Model file for the job. Use its own axes, mm. Face numbers are marked on the shaded views. A direction names the side the tool comes from. Coordinates: 2 decimals unless noted, no trailing zeros. Order: outer loops, then holes, each group sorted by start corner. A loop starts at its lowest first (then second) coordinate and runs counter-clockwise, first axis right, second up. Notation, with made-up numbers: (-40, 52) -> (12, 52) arc R32 cw to (12, 84) -> close; hole circle Ø7 at (13, -5). An arc over 180 degrees is marked (long way). Write item = value, one per line. Start each with the question number.
Q1. Flat gauge pins, fed straight in: pin 1 (1 mm diameter, centred on x = 1.07, y = -7.26, fed in from +Z); pin 2 (1.5 mm diameter, centred on y = -35.5, z = -5.5, fed in from -X); pin 3 (2 mm diameter, centred on y = -36, z = -13, fed in from +X); pin 4 (2.5 mm diameter, centred on x = 4, y = -40, fed in from +Z). Where does each tip first touch, or does it go through?
Q2. Cut at D-D, the plane x = -1.75. List the corners of the cut face in (y, z), plus the area to 3 significant figures.
Q3. Cut at C-C, the plane y = -31.5. List the corners of the cut face in (x, z), plus the area to 4 significant figures.
Q4. Cut at B-B, the plane z = -11.75. List the corners of the cut face in (x, y), plus the area to 3 significant figures.
Q5. Cut at A-A, the plane z = -3. List the corners of the cut face in (x, y), plus the area to 3 significant figures.
Q6. 3-axis set-ups, long thin cutter, end or side, ignore diameter. For the marked faces 1 and 2: which of +Z, -Z, +X, -X, +Y, -Y reach the whole face in a straight line?
Q7. Wall check: line 1 (X direction, y = -35.5, z = -6.25); line 2 (Y direction, x = 1, z = -3); line 3 (Y direction, x = 3.75, z = -13.5). Give the ranges that are in metal, low to high. Write a range as from..to.
from build123d import *

# Parameters (mm, degrees)
EXTRUDE_START                = -2
EXTRUDE_1_DEPTH              = 13
SKETCH_2_R                   = 11
CUT_EXTRUDE_1_DEPTH          = 5
SKETCH_3_R                   = 1.5
EXTRUDE_2_DEPTH              = 2
EXTRUDE_3_DEPTH              = 2
HOLE_WIZARD_M2_4_D           = 1.6
HOLE_WIZARD_M2_4_DEPTH       = 5.2
HOLE_WIZARD_M2_4_CSINK_D     = 2.05
HOLE_WIZARD_M2_4_CSINK_ANGLE = 90
HOLE_WIZARD_M2_4_TIP         = 0.480688495
HOLE_WIZARD_M2_5_D           = 1.6
HOLE_WIZARD_M2_5_DEPTH       = 5.2
HOLE_WIZARD_M2_5_CSINK_D     = 2.05
HOLE_WIZARD_M2_5_CSINK_ANGLE = 90
HOLE_WIZARD_M2_5_TIP         = 0.480688495


with BuildPart() as part:
    # 草图1 → 凸台-拉伸1 (new body)
    with BuildSketch(Plane.XY.offset(EXTRUDE_START)):
        with BuildLine():
            Line((2.570888862, -12.45291013), (-3.464101615, -2))
            Line((-3.464101615, -2), (-5.196152423, -3))
            Line((-5.196152423, -3), (1.320888862, -14.287846621))
            Line((1.320888862, -14.287846621), (1.320888862, -44.355557574))
            ThreePointArc((1.320888862, -44.355557574), (1.933218512, -44.007523283), (2.570888862, -43.708438024))
            Line((2.570888862, -43.708438024), (2.570888862, -12.45291013))
        make_face()
    extrude(amount=-EXTRUDE_1_DEPTH)

    # 草图2 → 切除-拉伸1 (cut)
    with BuildSketch(Plane(origin=(0, 0, -15), x_dir=(-1, 0, 0), z_dir=(0, 0, -1))):
        with Locations((-6.070888862, -52)):
            Circle(SKETCH_2_R)
    extrude(amount=-CUT_EXTRUDE_1_DEPTH, mode=Mode.SUBTRACT)

    # 草图3 → 凸台-拉伸2 (add)
    with BuildSketch(Plane(origin=(0, 0, -15), x_dir=(-1, 0, 0), z_dir=(0, 0, -1))):
        with Locations((-4.070888862, -39.661037321)):
            Circle(SKETCH_3_R)
        with BuildLine():
            Line((-2.570888862, -41.571673193), (-2.570888862, -39.661037321))
            ThreePointArc((-2.570888862, -39.661037321), (-3.098777733, -40.803403266), (-4.310888798, -41.141712853))
            ThreePointArc((-4.310888798, -41.141712853), (-3.432117057, -41.321194666), (-2.570888862, -41.571673193))
        make_face()
        with BuildLine():
            Line((-2.570888862, -39.661037321), (-2.570888862, -38.161037321))
            Line((-2.570888862, -38.161037321), (-4.070888862, -38.161037321))
            ThreePointArc((-4.070888862, -38.161037321), (-3.010228691, -38.600377149), (-2.570888862, -39.661037321))
        make_face()
    extrude(amount=-EXTRUDE_2_DEPTH)

    # 草图4 → 凸台-拉伸3 (add)
    with BuildSketch(Plane.XY.offset(-2)):
        with BuildLine():
            Line((0.320888862, -8.555795813), (2.570888862, -12.45291013))
            Line((2.570888862, -12.45291013), (2.570888862, -7.256757708))
            ThreePointArc((2.570888862, -7.256757708), (1.820888862, -8.555795813), (0.320888862, -8.555795813))
        make_face()
        with BuildLine():
            ThreePointArc((0.320888862, -8.555795813), (1.820888862, -8.555795813), (2.570888862, -7.256757708))
            Line((2.570888862, -7.256757708), (-0.429111138, -7.256757708))
            Line((-0.429111138, -7.256757708), (0.320888862, -8.555795813))
        make_face()
        with BuildLine():
            Line((-0.429111138, -7.256757708), (2.570888862, -7.256757708))
            ThreePointArc((2.570888862, -7.256757708), (1.070888862, -5.756757708), (-0.429111138, -7.256757708))
        make_face()
    extrude(amount=-EXTRUDE_3_DEPTH)

    # M2 螺纹孔4
    with Locations(Plane.XY.offset(-2)):
        with Locations((1.070888862, -7.256757708)):
            CounterSinkHole(HOLE_WIZARD_M2_4_D / 2, HOLE_WIZARD_M2_4_CSINK_D / 2, depth=HOLE_WIZARD_M2_4_DEPTH, counter_sink_angle=HOLE_WIZARD_M2_4_CSINK_ANGLE)
            with Locations((0, 0, -(HOLE_WIZARD_M2_4_DEPTH + HOLE_WIZARD_M2_4_TIP / 2))):  # 118° drill point
                Cone(0, HOLE_WIZARD_M2_4_D / 2, HOLE_WIZARD_M2_4_TIP, mode=Mode.SUBTRACT)

    # M2 螺纹孔5
    with Locations(Plane(origin=(0, 0, -15), x_dir=(-1, 0, 0), z_dir=(0, 0, -1))):
        with Locations((-4.070888862, -39.661037321)):
            CounterSinkHole(HOLE_WIZARD_M2_5_D / 2, HOLE_WIZARD_M2_5_CSINK_D / 2, depth=HOLE_WIZARD_M2_5_DEPTH, counter_sink_angle=HOLE_WIZARD_M2_5_CSINK_ANGLE)
            with Locations((0, 0, -(HOLE_WIZARD_M2_5_DEPTH + HOLE_WIZARD_M2_5_TIP / 2))):  # 118° drill point
                Cone(0, HOLE_WIZARD_M2_5_D / 2, HOLE_WIZARD_M2_5_TIP, mode=Mode.SUBTRACT)


solid = part.part
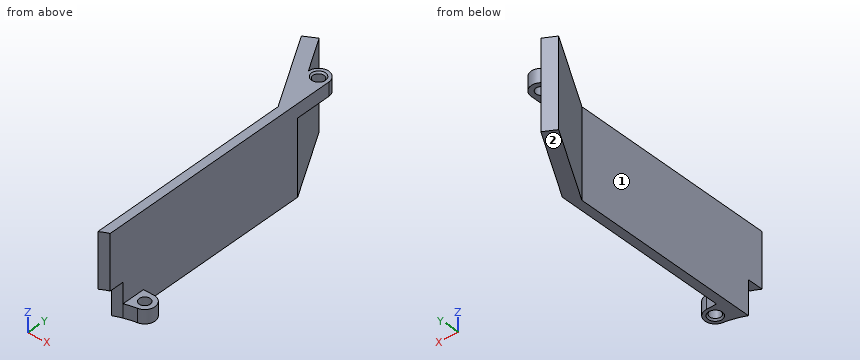
Here are the results:
q1.pin_1 = through
q1.pin_2 = 1.32
q1.pin_3 = 2.57
q1.pin_4 = -13
q2.outline = (-8.97, -15) -> (-4.97, -15) -> (-4.97, -2) -> (-8.97, -2) -> close
q2.area = 52.0 mm²
q3.outline = (1.32, -15) -> (2.57, -15) -> (2.57, -2) -> (1.32, -2) -> close
q3.area = 16.25 mm²
q4.outline = (-5.2, -3) -> (1.32, -14.29) -> (1.32, -42.08) arc R11 cw to (2.57, -41.57) -> (2.57, -12.45) -> (-3.46, -2) -> close
q4.area = 60.7 mm²
q5.outline = (-5.2, -3) -> (1.32, -14.29) -> (1.32, -44.36) arc R9 cw to (2.57, -43.71) -> (2.57, -7.26) arc R1.5 ccw to (-0.43, -7.26) -> (-3.46, -2) -> close; hole circle Ø1.6 at (1.07, -7.26)
q5.area = 72.7 mm²
q6.face_1 = +Z, -Z, -X, -Y
q6.face_2 = -Z, +X, -X, +Y, -Y
q7.line_1 = 1.32..2.57
q7.line_2 = -13.73..-8.05, -6.46..-5.76
q7.line_3 = -41.25..-40.39, -38.93..-38.16
